Geometry: see drawing. Coordinates: mm, zero at the bounding-box minimum. A direction names the side the tool comes from. Round coordinates to 2 decimals unless told otherwise and drop trailing zeros. Loops run counter-clockwise (first coordinate to the right, second up) from the corner with the lowest first, then second, coordinate; pieces in that order, holes last. Notation, with made-up numbers: (67.5, 76) - (104.5, 76) arc R12 ccw to (104.5, 96) - close; hole circle Ø3 at (4, 16). An arc over 180 degrees is marked (long way). Use CSV: the item, a comma, the result in double quotes. Start each with the question number.
1. Cut plane A-A (y = 22). Return loops of the section in (x, z), and give its area (3 significant figures).
2. Cut plane D-D (z = 27.5). Return loops of the section in (x, y), and give its area (3 significant figures).
3. Cut plane C-C (y = 36.5). Return loops of the section in (x, z).
4. Pin query (flat end, axial travel): P1, Ø11.5, axis at x = 69.5, y = 21.5, coming from the -Z side; P2, Ø19, axis at x = 72, y = 22.5, coming from the +Z side; P3, Ø6.5, axis at y = 17.5, z = 4, coming from the +X side. Return the tip coordinate at first contact, or that it passes through.
5. Access query for the marked faces 1, 2 and 3. Directions: +Z, -Z, +X, -X, +Y, -Y. A direction counts if a zero-diameter tool reaches every point of the face in a straight line with its end or side. Return the directions, or none.
6. Cut plane B-B (x = 72.5). Return loops of the section in (y, z).
7. Material intervals for probe 1 along Y at (x, z) = (55.5, 21); probe 2 along Z at (x, y) = (40.5, 9); probe 3 along X at (y, z) = (13.5, 10), sorted ascending. Write a range as from..to.
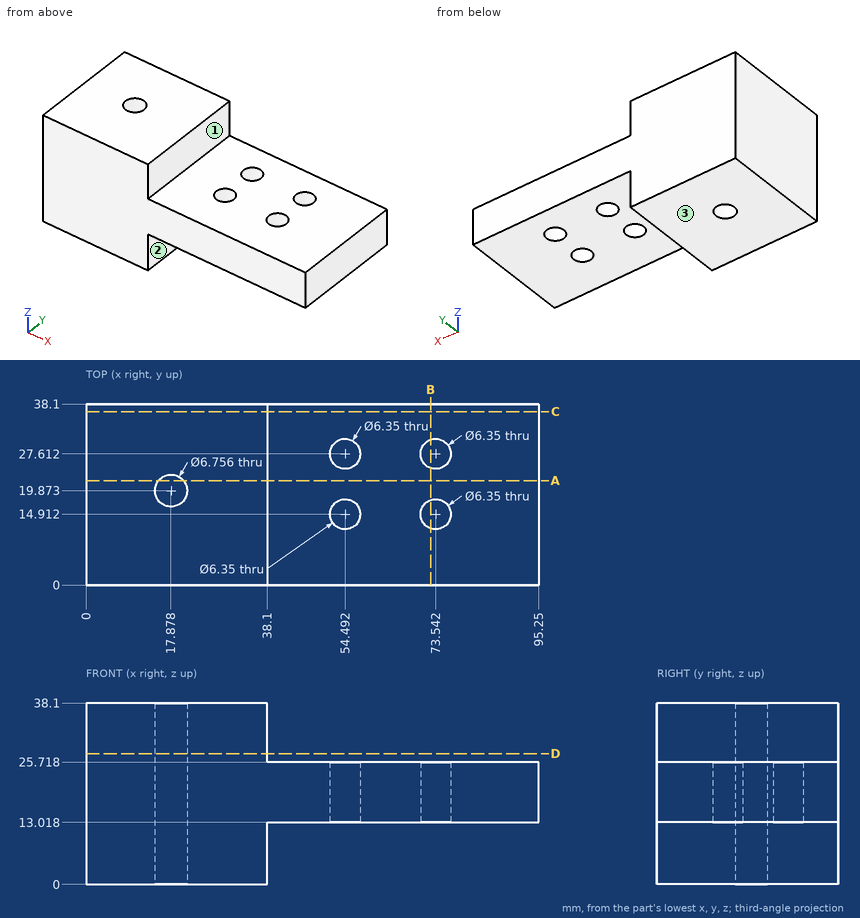
Established:
1,outline,"(0, 0) - (15.25, 0) - (15.25, 38.1) - (0, 38.1) - close; (20.5, 0) - (38.1, 0) - (38.1, 13.02) - (95.25, 13.02) - (95.25, 25.72) - (38.1, 25.72) - (38.1, 38.1) - (20.5, 38.1) - close"
1,area,"1,980 mm2"
2,outline,"(0, 0) - (38.1, 0) - (38.1, 38.1) - (0, 38.1) - close; hole circle Ø6.76 at (17.88, 19.87)"
2,area,"1,420 mm2"
3,outline,"(0, 0) - (38.1, 0) - (38.1, 13.02) - (95.25, 13.02) - (95.25, 25.72) - (38.1, 25.72) - (38.1, 38.1) - (0, 38.1) - close"
4,P1,"stops at z = 13.02"
4,P2,"stops at z = 25.72"
4,P3,"stops at x = 38.1"
5,face 1,"+Z, +X, +Y, -Y"
5,face 2,"-Z, +X, +Y, -Y"
5,face 3,"-Z, +X, -X, +Y, -Y"
6,outline,"(0, 13.02) - (11.91, 13.02) - (11.91, 25.72) - (0, 25.72) - close; (17.91, 13.02) - (24.61, 13.02) - (24.61, 25.72) - (17.91, 25.72) - close; (30.61, 13.02) - (38.1, 13.02) - (38.1, 25.72) - (30.61, 25.72) - close"
7,probe 1,"y = 0..11.9, 17.92..24.6, 30.62..38.1"
7,probe 2,"z = 13.02..25.72"
7,probe 3,"x = 0..38.1"
